from build123d import *

# Parameters (mm, degrees)
SKETCH1_W           = 20.5
SKETCH1_H           = 20.5
BOSS_EXTRUDE1_DEPTH = 1.5
CUT_EXTRUDE1_START  = 1.5
SKETCH2_R           = 0.75
CUT_EXTRUDE1_DEPTH  = 2.5
BOSS_EXTRUDE2_START = 1.5
SKETCH3_W           = 15
SKETCH3_H           = 14.5
BOSS_EXTRUDE2_DEPTH = 2


with BuildPart() as part:
    # Sketch1 → Boss-Extrude1 (new body)
    with BuildSketch(Plane(origin=(0, 0, 0), x_dir=(1, 0, 0), z_dir=(0, 1, 0))):
        Rectangle(SKETCH1_W, SKETCH1_H)
    extrude(amount=BOSS_EXTRUDE1_DEPTH)

    # Sketch2 → Cut-Extrude1 (cut, through all)
    with BuildSketch(Plane(origin=(0, 0, 0), x_dir=(1, 0, 0), z_dir=(0, 1, 0)).offset(CUT_EXTRUDE1_START)):
        with Locations((-9, 8.95)):
            Circle(SKETCH2_R)
        with Locations((-9, 6.41)):
            Circle(SKETCH2_R)
        with Locations((-9, 3.87)):
            Circle(SKETCH2_R)
        with Locations((-9, 1.33)):
            Circle(SKETCH2_R)
        with Locations((-9, -1.21)):
            Circle(SKETCH2_R)
        with Locations((-9, -3.75)):
            Circle(SKETCH2_R)
        with Locations((-9, -6.29)):
            Circle(SKETCH2_R)
        with Locations((-9, -8.83)):
            Circle(SKETCH2_R)
        with Locations((9, -8.83)):
            Circle(SKETCH2_R)
        with Locations((9, -6.29)):
            Circle(SKETCH2_R)
        with Locations((9, -3.75)):
            Circle(SKETCH2_R)
        with Locations((9, -1.21)):
            Circle(SKETCH2_R)
        with Locations((9, 1.33)):
            Circle(SKETCH2_R)
        with Locations((9, 3.87)):
            Circle(SKETCH2_R)
        with Locations((9, 6.41)):
            Circle(SKETCH2_R)
        with Locations((9, 8.95)):
            Circle(SKETCH2_R)
    extrude(amount=-CUT_EXTRUDE1_DEPTH, mode=Mode.SUBTRACT)

    # Sketch3 → Boss-Extrude2 (add)
    with BuildSketch(Plane(origin=(0, 0, 0), x_dir=(1, 0, 0), z_dir=(0, 1, 0)).offset(BOSS_EXTRUDE2_START)):
        with Locations((0, -2.5)):
            Rectangle(SKETCH3_W, SKETCH3_H)
    extrude(amount=BOSS_EXTRUDE2_DEPTH)


solid = part.part
CAD build for the part. Positions are in the model's coordinates, mm. A direction names the side the tool comes from. Give positions to 0.01 mm unless a question says otherwise; leave off trailing zeros. Order: outer loops, then holes, each group sorted by start corner. A loop starts at its lowest first (then second) coordinate and runs counter-clockwise, first axis right, second up. Notation, with made-up numbers: (43, 50.5) - (85, 50.5) arc R24 cw to (85, 67.5) - close; hole circle Ø5 at (-3.75, 12.5). An arc over 180 degrees is marked (long way). Answer in a Markdown table with one row per item.
1. Flat gauge pins, fed straight in: pin 1 (2.5 mm diameter, centred on x = 9, z = -6.41, fed in from +Y); pin 2 (0.9 mm diameter, centred on x = 9, z = 8.83, fed in from +Y); pin 3 (0.6 mm diameter, centred on y = 2.5, z = 2.5, fed in from +X). Where does each tip first touch, or does it go through?
Data:
| item | result |
|---|---|
| pin 1 | stops at y = 1.5 |
| pin 2 | passes through |
| pin 3 | stops at x = 7.5 |
2. Tool access for faces 5 (the flat face through (7.5, 2, 3)), 6 (the cylindrical face through (8.25, 0.76, 1.18)): list every direction of +Z, -Z, +X, -X, +Y, -Y with a clear straight run to the whole face (end or side of a thin tool).
Data:
| item | result |
|---|---|
| face 5 | +Z, -Z, +X, +Y |
| face 6 | +Y, -Y |
3. Pull direction Z, two halves, no side cores. Call faces 1 (the flat face through (-7.5, 2, 3)), 2 (the cylindrical face through (-9.75, 0.76, 6.26)), 3 (the cylindrical face through (8.25, 0.76, -3.9)), 4 (the flat face through (0, 1, 10.25)): pulls with the +Z half, pulls with the -Z half, needs draft (parallel to the pull), parting line crosses it, or undercut.
Data:
| item | result |
|---|---|
| face 1 | needs draft |
| face 2 | undercut |
| face 3 | undercut |
| face 4 | pulls with the +Z half |
4. Saw through at C-C, the plane x = -6.75. Give the cut face in (y, z).
Data:
| item | result |
|---|---|
| outline | (0, -10.25) - (1.5, -10.25) - (1.5, -4.75) - (3.5, -4.75) - (3.5, 9.75) - (1.5, 9.75) - (1.5, 10.25) - (0, 10.25) - close |
5. Saw through at D-D, the plane z = -0.25. Give the cut face in (x, y), plus the area to 4 significant figures.
Data:
| item | result |
|---|---|
| outline | (-10.25, 0) - (10.25, 0) - (10.25, 1.5) - (7.5, 1.5) - (7.5, 3.5) - (-7.5, 3.5) - (-7.5, 1.5) - (-10.25, 1.5) - close |
| area | 60.75 mm² |
6. Saw through at B-B, the plane y = 0.4. Count the separate pieces of the cut face and the enclosed holes in it, plus the area to 3 significant figures.
Data:
| item | result |
|---|---|
| separate pieces | 1 |
| enclosed holes | 16 |
| area | 392 mm² |
7. Saw through at A-A, the plane z = -8.95. Give the cut face in (x, y).
Data:
| item | result |
|---|---|
| outline | (-10.25, 0) - (-9.75, 0) - (-9.75, 1.5) - (-10.25, 1.5) - close; (-8.25, 0) - (8.25, 0) - (8.25, 1.5) - (-8.25, 1.5) - close; (9.75, 0) - (10.25, 0) - (10.25, 1.5) - (9.75, 1.5) - close |
8. Probe probe 1 along X at (y, z) = (0.85, -3.87); probe 2 along Z at (x, y) = (2.5, 2.4); probe 3 along Y at (x, z) = (7.5, -9). List the from-to ranges inside material, lowest first. Write a range as [from, to].
Data:
| item | result |
|---|---|
| probe 1 | x = [-10.25, -9.75], [-8.25, 8.25], [9.75, 10.25] |
| probe 2 | z = [-4.75, 9.75] |
| probe 3 | y = [0, 1.5] |
